Can you work these out from the model? Positions are in its coordinate system, mm. A direction names the side the tool comes from. Give positions to 0.01 mm unless a question says otherwise; leave off trailing zeros. Order: outer loops, then holes, each group sorted by start corner. A loop starts at its lowest first (then second) coordinate and runs counter-clockwise, first axis right, second up. Notation, with made-up numbers: (54, 6) - (67, 6) arc R23 cw to (67, 16) - close; hole circle Ø9 at (20.5, 55). An arc over 180 degrees is marked (long way). Answer as CSV lines item,"result".
```python
from build123d import *

# Parameters (mm, degrees)
CROQUIS1_R              = 9
CROQUIS1_R_2            = 6
SALIENTE_EXTRUIR1_DEPTH = 10
CORTAR_EXTRUIR1_DEPTH   = 17.186414056
SALIENTE_EXTRUIR2_START = -10
SALIENTE_EXTRUIR2_DEPTH = 10
REDONDEO1_R             = 5
CROQUIS4_R              = 1.625
CORTAR_EXTRUIR2_DEPTH   = 26.698219636
CORTAR_EXTRUIR4_DEPTH   = 22.659835929
CROQUIS6_R              = 5.5
CORTAR_EXTRUIR5_DEPTH   = 2.5
CORTAR_EXTRUIR6_DEPTH   = 2.3


with BuildPart() as part:
    # Croquis1 → Saliente-Extruir1 (new body)
    with BuildSketch(Plane.XY):
        Circle(CROQUIS1_R)
        Circle(CROQUIS1_R_2, mode=Mode.SUBTRACT)
    extrude(amount=SALIENTE_EXTRUIR1_DEPTH)

    # Croquis2 → Cortar-Extruir1 (cut, through all)
    with BuildSketch(Plane.XY.offset(10)):
        with BuildLine():
            Line((0, 0), (8.923003752, 1.17473573))
            ThreePointArc((8.923003752, 1.17473573), (9, 0), (8.923003752, -1.17473573))
            Line((8.923003752, -1.17473573), (0, 0))
        make_face()
    extrude(amount=-CORTAR_EXTRUIR1_DEPTH, mode=Mode.SUBTRACT)

    # Croquis3 → Saliente-Extruir2 (add)
    with BuildSketch(Plane.XY.offset(10).offset(SALIENTE_EXTRUIR2_START)):
        with BuildLine():
            Line((-4.974937186, 7.5), (-16.974937186, 7.5))
            Line((-16.974937186, 7.5), (-16.974937186, -7.5))
            Line((-16.974937186, -7.5), (-4.974937186, -7.5))
            ThreePointArc((-4.974937186, -7.5), (-9, 0), (-4.974937186, 7.5))
        make_face()
    extrude(amount=SALIENTE_EXTRUIR2_DEPTH)

    # Redondeo1
    redondeo1_edges = [part.edges().sort_by_distance(p)[0] for p in [
        (-16.974937186, 0, 0),
        (-16.974937186, 0, 10),
    ]]
    fillet(redondeo1_edges, radius=REDONDEO1_R - 0.0001)  # a hair under: the kernel refuses the full size

    # Croquis4 → Cortar-Extruir2 (cut, through all)
    with BuildSketch(Plane.XZ.offset(7.5)):
        with Locations((-11.974937186, 5)):
            Circle(CROQUIS4_R)
    extrude(amount=-CORTAR_EXTRUIR2_DEPTH, mode=Mode.SUBTRACT)

    # Croquis5 → Cortar-Extruir4 (cut, through all)
    with BuildSketch(Plane.XY.offset(10)):
        with BuildLine():
            Line((-8.645808233, 2.5), (-21.808614769, 2.5))
            Line((-21.808614769, 2.5), (-21.808614769, -2.5))
            Line((-21.808614769, -2.5), (-8.645808233, -2.5))
            ThreePointArc((-8.645808233, -2.5), (-9, 0), (-8.645808233, 2.5))
        make_face()
    extrude(amount=-CORTAR_EXTRUIR4_DEPTH, mode=Mode.SUBTRACT)

    # Croquis6 → Cortar-Extruir5 (cut, symmetric)
    with BuildSketch(Plane(origin=(0, 0, 0), x_dir=(1, 0, 0), z_dir=(0, 1, 0))):
        with Locations((-11.974937186, -5)):
            Circle(CROQUIS6_R)
    extrude(amount=CORTAR_EXTRUIR5_DEPTH, both=True, mode=Mode.SUBTRACT)

    # Croquis7 → Cortar-Extruir6 (cut)
    with BuildSketch(Plane.XZ.offset(7.5)):
        Polygon((-8.799510705, 5), (-10.387223945, 7.75), (-13.562650426, 7.75), (-15.150363666, 5), (-13.562650426, 2.25), (-10.387223945, 2.25), align=None)
    extrude(amount=-CORTAR_EXTRUIR6_DEPTH, mode=Mode.SUBTRACT)


solid = part.part
```
1) I'm going to push flat-ended pins straight in: P1, Ø5, axis at x = 1, z = 6, coming from the -Y side; P2, Ø1.5, axis at x = -2.5, z = 7.5, coming from the +Y side; P3, Ø5, axis at x = -10, z = 5.5, coming from the +Y side; P4, Ø3, axis at x = -12, z = 5, coming from the -Y side. Where does each tip first touch, or does it pass through?
Answer block:
P1,"y = -9"
P2,"y = 8.83"
P3,"y = 7.5"
P4,"through"
2) I want a section at A-A on x = 0. Write out the boundary of the cut face in (y, z).
Answer block:
outline,"(-9, 0) - (-6, 0) - (-6, 10) - (-9, 10) - close; (6, 0) - (9, 0) - (9, 10) - (6, 10) - close"
3) Which directions (+Z, -Z, +X, -X, +Y, -Y) give clear straight access to the entire face, cutting with the end or side of a thin tool? Please do faces 5 (the flat face through (-10, 7.5, 5)), 6 (the flat face through (-10, 2.5, 6)), 7 (the flat face through (-12, -6, 2.25)).
Answer block:
face 5,"+Z, -Z, -X, +Y"
face 6,"-X"
face 7,"-Y"
4) I want a section at B-B on x = -11. Write out the boundary of the cut face in (y, z).
Answer block:
outline,"(-7.5, 0) - (-2.5, 0) - (-2.5, 3.7) - (-5.2, 3.7) - (-5.2, 2.25) - (-7.5, 2.25) - close; (-7.5, 7.75) - (-5.2, 7.75) - (-5.2, 6.3) - (-2.5, 6.3) - (-2.5, 10) - (-7.5, 10) - close; (2.5, 0) - (7.5, 0) - (7.5, 3.7) - (2.5, 3.7) - close; (2.5, 6.3) - (7.5, 6.3) - (7.5, 10) - (2.5, 10) - close"
5) If we mould it in two halves opening along Z, with no side actions, what happens to faces 1 (the cylindrical face through (-6.475, 0.035, 5.077)), 2 (the flat face through (-6.3, 0.1, 0)), 3 (the flat face through (7.415, 0.976, 5.07)), 4 (the cylindrical face through (-13.6, -3.87, 5.07))? For each: +Z half, -Z half, draft (parallel to the pull), parting line (faces both ways), or undercut.
Answer block:
face 1,"undercut"
face 2,"-Z half"
face 3,"draft"
face 4,"undercut"
6) I want a section at D-D on y = 0. Write out the boundary of the cut face in (x, z), plus the area to 3 significant figures.
Answer block:
outline,"(-9, 0) - (-6, 0) - (-6, 10) - (-9, 10) - (-9, 9.63) arc R5.5 cw to (-9, 0.37) - close"
area,"13.5 mm2"
7) I need wall thicknesses on line 1 along Y through (x, z) = (-8, 7); line 2 along Y through (x, z) = (0, 5); line 3 along X through (y, z) = (5.25, 4). Which ranges of each line are inside material? Lowest first, please. Write a range as [from, to].
Answer block:
line 1,"[-7.5, -2.5], [2.5, 7.5]"
line 2,"[-9, -6], [6, 9]"
line 3,"[-16.87, -13.26], [-10.69, -2.9], [2.9, 7.31]"
8) I want a section at C-C on z = 4. Write out the boundary of the cut face in (x, y), plus the area to 3 significant figures.
Answer block:
outline,"(-16.87, -7.5) - (-14.57, -7.5) - (-14.57, -5.2) - (-13.26, -5.2) - (-13.26, -2.5) - (-16.87, -2.5) - close; (-16.87, 2.5) - (-13.26, 2.5) - (-13.26, 7.5) - (-16.87, 7.5) - close; (-10.69, -5.2) - (-9.38, -5.2) - (-9.38, -7.5) - (-4.97, -7.5) arc R9 ccw to (8.92, -1.17) - (5.95, -0.78) arc R6 cw (long way) to (5.95, 0.78) - (8.92, 1.17) arc R9 ccw to (-4.97, 7.5) - (-10.69, 7.5) - (-10.69, 2.5) - (-6.57, 2.5) - (-6.57, -2.5) - (-10.69, -2.5) - close"
area,"188 mm2"
